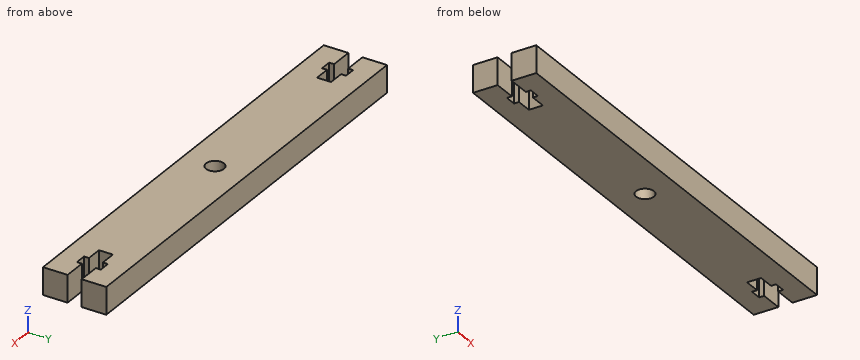
```python
from build123d import *

# Parameters (mm, degrees)
F0_W     = 98.8
F0_H     = 14
F1_DEPTH = 6
F2_W     = 5
F2_H     = 3.1
F2_W_2   = 2.5
F2_H_2   = 1.1
F2_W_3   = 3.5
F3_DEPTH = 6
F4_R     = 1.975
F5_DEPTH = 6


with BuildPart() as f1:
    # F0 (on Top) → F1 (new body)
    with BuildSketch(Plane.XY):
        Rectangle(F0_W, F0_H)
    extrude(amount=F1_DEPTH)

    # F2 (on face) → F3 (cut, through all)
    with BuildSketch(Plane.XY.offset(6)):
        with Locations((-46.9, 0)):
            Rectangle(F2_W, F2_H)
        with Locations((-43.15, 0)):
            Rectangle(F2_W_2, F2_H)
        with Locations((-43.15, -2.1)):
            Rectangle(F2_W_2, F2_H_2)
        with Locations((-40.15, 0)):
            Rectangle(F2_W_3, F2_H)
        with Locations((-43.15, 2.1)):
            Rectangle(F2_W_2, F2_H_2)
        with Locations((46.9, 0)):
            Rectangle(F2_W, F2_H)
        with Locations((43.15, 0)):
            Rectangle(F2_W_2, F2_H)
        with Locations((43.15, -2.1)):
            Rectangle(F2_W_2, F2_H_2)
        with Locations((43.15, 2.1)):
            Rectangle(F2_W_2, F2_H_2)
        with Locations((40.15, 0)):
            Rectangle(F2_W_3, F2_H)
    extrude(amount=-F3_DEPTH, mode=Mode.SUBTRACT)

    # F4 (on face) → F5 (cut, through all)
    with BuildSketch(Plane.XY.offset(6)):
        Circle(F4_R)
    extrude(amount=-F5_DEPTH, mode=Mode.SUBTRACT)


solid = f1.part
```
CAD build for the part. Positions are in the model's coordinates, mm. Round coordinates to 2 decimals unless told otherwise and drop trailing zeros. Write each loop counter-clockwise with the first axis right and the second up, starting at its lowest first coordinate (ties: lowest second). Pieces come first, ordered by that corner, then holes. Notation, with made-up numbers: (38.25, 60) - (90.25, 60) arc R16 ccw to (90.25, 88) - close; hole circle Ø11 at (9.25, -26). An arc over 180 degrees is marked (long way). Return JSON: item names as keys, results as strings. Group by question number.
Item 1: Probe probe 1 along X at (y, z) = (-2.25, 1.25); probe 2 along Y at (x, z) = (0, 1.45) (3 decimals); probe 3 along Y at (x, z) = (-45, 4.7). List the from-to ranges inside material, lowest first.
Item 2: Band-saw the part on A-A on y = 0. List the corners of the cut face in (x, z) (3 decimals), plus the area to 3 significant figures.
Item 3: Band-saw the part on B-B on x = 0. List the corners of the cut face in (y, z) (3 decimals), plus the area to 3 significant figures.
Resolved:
{
 "1": {"probe 1": "x = -49.4 to -44.4, -41.9 to 41.9, 44.4 to 49.4", "probe 2": "y = -7 to -1.975, 1.975 to 7", "probe 3": "y = -7 to -1.55, 1.55 to 7"},
 "2": {"outline": "(-38.4, 0) - (-1.975, 0) - (-1.975, 6) - (-38.4, 6) - close; (1.975, 0) - (38.4, 0) - (38.4, 6) - (1.975, 6) - close", "area": "437 mm²"},
 "3": {"outline": "(-7, 0) - (-1.975, 0) - (-1.975, 6) - (-7, 6) - close; (1.975, 0) - (7, 0) - (7, 6) - (1.975, 6) - close", "area": "60.3 mm²"}
}
